The model under review builds one solid part; all positions refer to its coordinate system, in mm. Coordinates: 2 decimals unless noted, no trailing zeros. Order: outer loops, then holes, each group sorted by start corner. A loop starts at its lowest first (then second) coordinate and runs counter-clockwise, first axis right, second up. Notation, with made-up numbers: (51.5, 23) - (73.5, 23) arc R19 ccw to (73.5, 45) - close; hole circle Ø1 at (38.25, 71.5). An arc over 180 degrees is marked (long way). Answer in a Markdown table with one row per item.
```python
from build123d import *

# Parameters (mm, degrees)
F0_W     = 660.4
F0_H     = 101.6
F1_DEPTH = 19.05
F2_SIZE  = 19.04999


# Not quite as in the source:
# - a fillet or chamfer is up to 0.001 mm smaller than in the source, because OpenCascade refuses the exact size


with BuildPart() as f1:
    # F0 (on Right) → F1 (new body)
    with BuildSketch(Plane.YZ):
        with Locations((330.2, 50.8)):
            Rectangle(F0_W, F0_H)
    extrude(amount=F1_DEPTH)

    # F2 (size 19.05 in the source; OpenCascade refuses exactly that, so slightly less here)
    f2_edges = [f1.edges().sort_by_distance(p)[0] for p in [
        (0, 330.2, 101.6),
        (0, 330.2, 0),
    ]]
    chamfer(f2_edges, length=F2_SIZE)


solid = f1.part
```
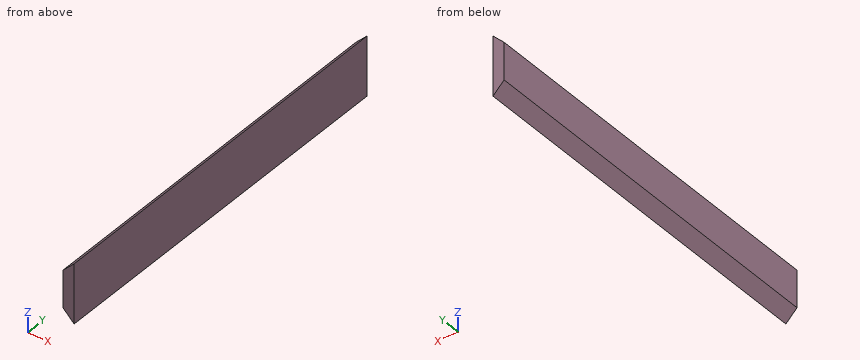
Item 1: We need section C-C, the plane z = 90. Write out the cut boundary in (x, y).
Check values:
| item | result |
|---|---|
| outline | (7.45, 0) - (19.05, 0) - (19.05, 660.4) - (7.45, 660.4) - close |
Item 2: We need section B-B, the plane x = 14. Write out the cut boundary in (y, z), then the cut area to 3 significant figures.
Check values:
| item | result |
|---|---|
| outline | (0, 5.05) - (660.4, 5.05) - (660.4, 96.55) - (0, 96.55) - close |
| area | 60,400 mm^2 |
Item 3: To check wall thickness, follow line 1 (Z direction, x = 12.25, y = 519.5); line 2 (Z direction, x = 18.25, y = 125); line 3 (X direction, y = 56, z = 6.5). State the ranges of each line that lie inside material, in increasing order. Write a range as from..to.
Check values:
| item | result |
|---|---|
| line 1 | 6.8..94.8 |
| line 2 | 0.8..100.8 |
| line 3 | 12.55..19.05 |
Item 4: Clearance check with flat-ended pins moving along their axes: pin 1 Ø1.5 at (x, y) = (17, 418.5) entering from -Z; pin 2 Ø2 at (x, y) = (17, 99.5) entering from -Z; pin 3 Ø1 at (x, y) = (9, 393) entering from -Z. State where each tip first meets the part, or that it passes through.
Check values:
| item | result |
|---|---|
| pin 1 | z = 1.3 |
| pin 2 | z = 1.05 |
| pin 3 | z = 9.55 |
